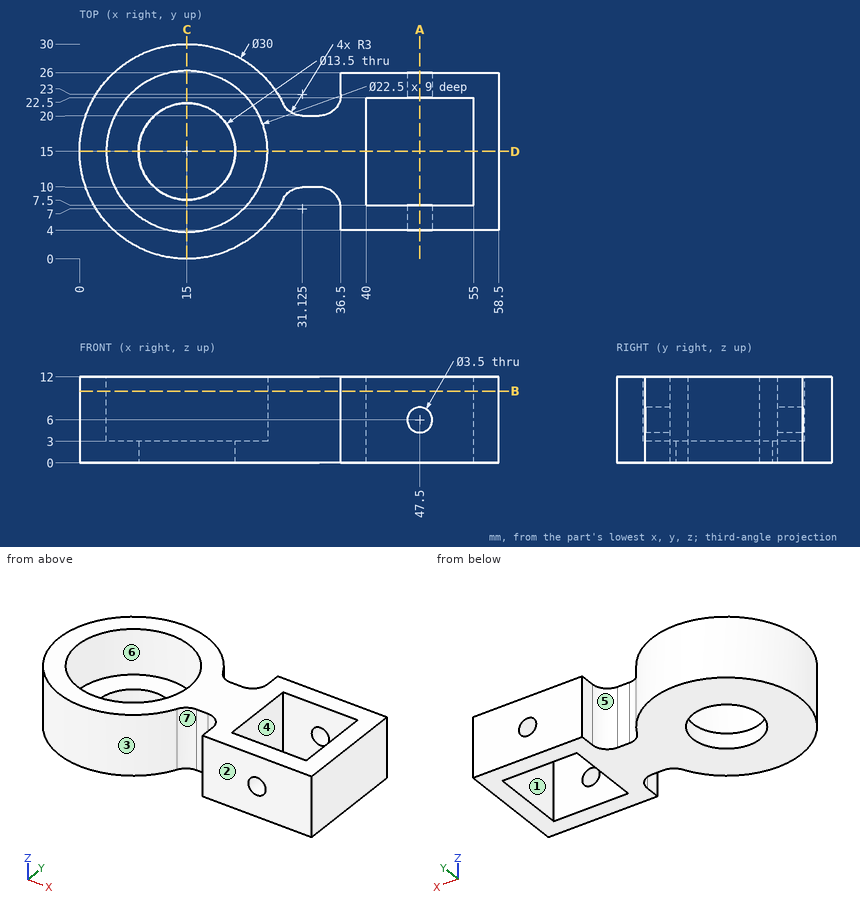
Can you work these out from the drawing? Everything is in mm from the part's minimum corner. A direction names the side the tool comes from. Give positions to 0.01 mm unless a question says otherwise; leave off trailing zeros. Order: outer loops, then holes, each group sorted by start corner. A loop starts at its lowest first (then second) coordinate and runs counter-clockwise, first axis right, second up. Notation, with made-up numbers: M -22,67 L 34,67 A26 ccw 34,91 Z; hole C -8.5,89 d5. An arc over 180 degrees is marked long. Use a Markdown table: item, result. Add a question column.
1. If we mould it in two halves opening along Y, with no side actions, what happens to the marked faces 1, 2 and 3? For each: +Y half, -Y half, draft (parallel to the pull), parting line (faces both ways), or undercut.
2. Suppose I cut it at D-D (y = 15). List the corners of the cut face in (x, z) for me, and give its area (3 significant figures).
3. Suppose I cut it at A-A (x = 47.5). List the corners of the cut face in (y, z) for me.
4. On a 3-axis mill with a long thin cutter (end or side, diameter ignored), from which of +Z, -Z, +X, -X, +Y, -Y can I reach the whole of each face in a straight line? I mean the marked faces 4, 5, 6 and 7. Say none if no direction works.
5. Suppose I cut it at B-B (z = 10). Give the number of separate pieces and of enclosed holes in the cut face.
6. I need wall thicknesses on probe 1 along X at (y, z) = (15.5, 11); probe 2 along Y at (x, z) = (15, 1.7); probe 3 along Y at (x, z) = (15, 8.5). Which ranges of each line are inside material? Lowest first, please. Write a range as from..to.
7. Suppose I cut it at C-C (x = 15). List the corners of the cut face in (y, z) for me, and give its area (3 significant figures).
8. For pin 1 Ø2.5 at (y, z) = (5.5, 8.5) entering from -X; pin 2 Ø11 at (x, y) = (10.5, 20) entering from +Z; pin 3 Ø4.5 at (x, z) = (47.5, 6) entering from -Y; pin 4 Ø3.5 at (x, z) = (51, 8.5) entering from +Y, each with a flat end and sliding along its axis, tell me the tip position at first contact or that it passes through.
Results list:
| question | item | result |
|---|---|---|
| 1 | face 1 | undercut |
| 1 | face 2 | -Y half |
| 1 | face 3 | parting line |
| 2 | outline | M 0,0 L 8.25,0 L 8.25,3 L 3.75,3 L 3.75,12 L 0,12 Z; M 21.75,0 L 40,0 L 40,12 L 26.25,12 L 26.25,3 L 21.75,3 Z; M 55,0 L 58.5,0 L 58.5,12 L 55,12 Z |
| 2 | area | 279 mm² |
| 3 | outline | M 4,0 L 7.5,0 L 7.5,4.25 L 4,4.25 Z; M 4,7.75 L 7.5,7.75 L 7.5,12 L 4,12 Z; M 22.5,0 L 26,0 L 26,4.25 L 22.5,4.25 Z; M 22.5,7.75 L 26,7.75 L 26,12 L 22.5,12 Z |
| 4 | face 4 | +Z, -Z |
| 4 | face 5 | +Z, -Z, +Y |
| 4 | face 6 | +Z |
| 4 | face 7 | +Z, -Z, -Y |
| 5 | separate pieces | 1 |
| 5 | enclosed holes | 2 |
| 6 | probe 1 | x = 0.01..3.76, 26.24..40, 55..58.5 |
| 6 | probe 2 | y = 0..8.25, 21.75..30 |
| 6 | probe 3 | y = 0..3.75, 26.25..30 |
| 7 | outline | M 0,0 L 8.25,0 L 8.25,3 L 3.75,3 L 3.75,12 L 0,12 Z; M 21.75,0 L 30,0 L 30,12 L 26.25,12 L 26.25,3 L 21.75,3 Z |
| 7 | area | 117 mm² |
| 8 | pin 1 | stops at x = 2.47 |
| 8 | pin 2 | stops at z = 12 |
| 8 | pin 3 | stops at y = 4 |
| 8 | pin 4 | stops at y = 26 |
